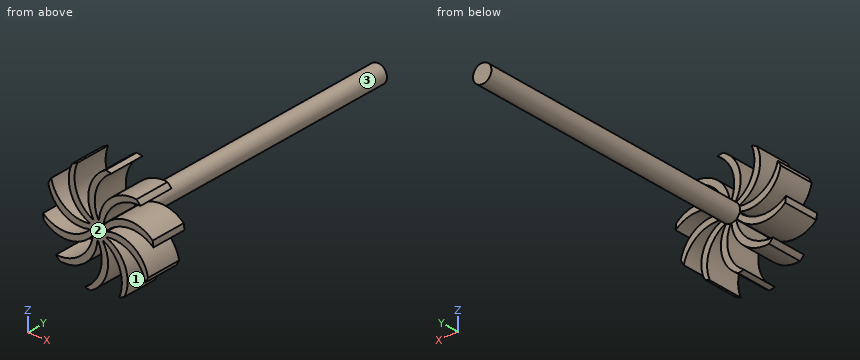
from build123d import *

# Parameters (mm, degrees)
F0_R     = 3.175
F1_DEPTH = 101.6
F3_DEPTH = 12.7


with BuildPart() as f1:
    # F0 (on Front) → F1 (new body)
    with BuildSketch(Plane.XZ):
        Circle(F0_R)
    extrude(amount=F1_DEPTH)

    # F2 (on face) → F3 (join)
    with BuildSketch(Plane.XZ.offset(101.6)):
        with BuildLine():
            ThreePointArc((0, 3.175), (-0.717894, 11.721662), (4.533669, 18.502658))
            ThreePointArc((4.533669, 18.502658), (3.549938, 18.716315), (2.556295, 18.877708))
            ThreePointArc((2.556295, 18.877708), (-3.036137, 11.70738), (-1.6328, 2.722974))
            ThreePointArc((-1.6328, 2.722974), (-0.847108, 3.059907), (0, 3.175))
        make_face()
        with BuildLine():
            ThreePointArc((1.866218, 2.568629), (6.309032, 9.904992), (14.543404, 12.304141))
            ThreePointArc((14.543404, 12.304141), (13.873134, 13.055215), (13.164125, 13.769834))
            ThreePointArc((13.164125, 13.769834), (4.425139, 11.256066), (0.279561, 3.162668))
            ThreePointArc((0.279561, 3.162668), (1.113244, 2.973434), (1.866218, 2.568629))
        make_face()
        with BuildLine():
            ThreePointArc((3.019604, 0.981129), (10.926122, 4.304951), (18.998054, 1.405861))
            ThreePointArc((18.998054, 1.405861), (18.897264, 2.407467), (18.743706, 3.402351))
            ThreePointArc((18.743706, 3.402351), (10.196162, 6.505317), (2.085139, 2.394331))
            ThreePointArc((2.085139, 2.394331), (2.648374, 1.751211), (3.019604, 0.981129))
        make_face()
        with BuildLine():
            ThreePointArc((16.196093, -10.029411), (16.703282, -9.159851), (17.163828, -8.264714))
            ThreePointArc((17.163828, -8.264714), (12.072598, -0.730242), (3.094265, 0.71144))
            ThreePointArc((3.094265, 0.71144), (3.154752, 0.358003), (3.175, 0))
            ThreePointArc((3.175, 0), (3.13591, -0.496679), (3.019604, -0.981129))
            ThreePointArc((3.019604, -0.981129), (11.369805, -2.939435), (16.196093, -10.029411))
        make_face()
        with BuildLine():
            ThreePointArc((-4.533669, -18.502658), (-3.549938, -18.716315), (-2.556295, -18.877708))
            ThreePointArc((-2.556295, -18.877708), (3.036137, -11.70738), (1.6328, -2.722974))
            ThreePointArc((1.6328, -2.722974), (0.847108, -3.059907), (0, -3.175))
            ThreePointArc((0, -3.175), (0.717894, -11.721662), (-4.533669, -18.502658))
        make_face()
        with BuildLine():
            ThreePointArc((7.207774, -17.633788), (8.129213, -17.228418), (9.027952, -16.774939))
            ThreePointArc((9.027952, -16.774939), (9.337711, -7.686873), (2.921487, -1.243196))
            ThreePointArc((2.921487, -1.243196), (2.483893, -1.9776), (1.866218, -2.568629))
            ThreePointArc((1.866218, -2.568629), (7.470609, -9.061056), (7.207774, -17.633788))
        make_face()
        with BuildLine():
            ThreePointArc((-14.543404, -12.304141), (-13.873134, -13.055215), (-13.164125, -13.769834))
            ThreePointArc((-13.164125, -13.769834), (-4.425139, -11.256066), (-0.279561, -3.162668))
            ThreePointArc((-0.279561, -3.162668), (-1.113244, -2.973434), (-1.866218, -2.568629))
            ThreePointArc((-1.866218, -2.568629), (-6.309032, -9.904992), (-14.543404, -12.304141))
        make_face()
        with BuildLine():
            ThreePointArc((-18.998054, -1.405861), (-18.897264, -2.407467), (-18.743706, -3.402351))
            ThreePointArc((-18.743706, -3.402351), (-10.196162, -6.505317), (-2.085139, -2.394331))
            ThreePointArc((-2.085139, -2.394331), (-2.648374, -1.751211), (-3.019604, -0.981129))
            ThreePointArc((-3.019604, -0.981129), (-10.926122, -4.304951), (-18.998054, -1.405861))
        make_face()
        with BuildLine():
            ThreePointArc((-3.019604, 0.981129), (-11.369805, 2.939435), (-16.196093, 10.029411))
            ThreePointArc((-16.196093, 10.029411), (-16.703282, 9.159851), (-17.163828, 8.264714))
            ThreePointArc((-17.163828, 8.264714), (-12.072598, 0.730242), (-3.094265, -0.71144))
            ThreePointArc((-3.094265, -0.71144), (-3.171916, 0.139916), (-3.019604, 0.981129))
        make_face()
        with BuildLine():
            ThreePointArc((-1.866218, 2.568629), (-7.470609, 9.061056), (-7.207774, 17.633788))
            ThreePointArc((-7.207774, 17.633788), (-8.129213, 17.228418), (-9.027952, 16.774939))
            ThreePointArc((-9.027952, 16.774939), (-9.337711, 7.686873), (-2.921487, 1.243196))
            ThreePointArc((-2.921487, 1.243196), (-2.483893, 1.9776), (-1.866218, 2.568629))
        make_face()
        with BuildLine():
            ThreePointArc((3.094265, 0.71144), (3.059907, 0.847108), (3.019604, 0.981129))
            ThreePointArc((3.019604, 0.981129), (2.648374, 1.751211), (2.085139, 2.394331))
            ThreePointArc((2.085139, 2.394331), (1.9776, 2.483893), (1.866218, 2.568629))
            ThreePointArc((1.866218, 2.568629), (1.113244, 2.973434), (0.279561, 3.162668))
            ThreePointArc((0.279561, 3.162668), (0.139916, 3.171916), (0, 3.175))
            ThreePointArc((0, 3.175), (-0.847108, 3.059907), (-1.6328, 2.722974))
            ThreePointArc((-1.6328, 2.722974), (-1.751211, 2.648374), (-1.866218, 2.568629))
            ThreePointArc((-1.866218, 2.568629), (-2.483893, 1.9776), (-2.921487, 1.243196))
            ThreePointArc((-2.921487, 1.243196), (-2.973434, 1.113244), (-3.019604, 0.981129))
            ThreePointArc((-3.019604, 0.981129), (-3.171916, 0.139916), (-3.094265, -0.71144))
            ThreePointArc((-3.094265, -0.71144), (-3.059907, -0.847108), (-3.019604, -0.981129))
            ThreePointArc((-3.019604, -0.981129), (-2.648374, -1.751211), (-2.085139, -2.394331))
            ThreePointArc((-2.085139, -2.394331), (-1.9776, -2.483893), (-1.866218, -2.568629))
            ThreePointArc((-1.866218, -2.568629), (-1.113244, -2.973434), (-0.279561, -3.162668))
            ThreePointArc((-0.279561, -3.162668), (-0.139916, -3.171916), (0, -3.175))
            ThreePointArc((0, -3.175), (0.847108, -3.059907), (1.6328, -2.722974))
            ThreePointArc((1.6328, -2.722974), (1.751211, -2.648374), (1.866218, -2.568629))
            ThreePointArc((1.866218, -2.568629), (2.483893, -1.9776), (2.921487, -1.243196))
            ThreePointArc((2.921487, -1.243196), (2.973434, -1.113244), (3.019604, -0.981129))
            ThreePointArc((3.019604, -0.981129), (3.13591, -0.496679), (3.175, 0))
            ThreePointArc((3.175, 0), (3.154752, 0.358003), (3.094265, 0.71144))
        make_face()
    extrude(amount=F3_DEPTH)


solid = f1.part
For this review, take the finished solid that the model builds, in its own axes (mm). Face numbers are marked on the shaded views. Round coordinates to 2 decimals unless told otherwise and drop trailing zeros. Loops run counter-clockwise (first coordinate to the right, second up) from the corner with the lowest first, then second, coordinate; pieces in that order, holes last. Notation, with made-up numbers: (82, 31.25) - (97, 31.25) arc R12 cw to (97, 50.25) - close; hole circle Ø7 at (20.25, 15). An arc over 180 degrees is marked (long way). Use one line per item in the form item = value.
Item 1: Mouldability with a two-part tool opening along X and no side actions: class the marked faces 1, 2 and 3 as +X half, -X half, draft (parallel to the pull), parting line (faces both ways), or undercut.
Answers:
face_1 = undercut
face_2 = draft
face_3 = parting line
Item 2: For line 1 (Y direction, x = 0, z = 15); line 2 (X direction, y = -104.5, z = 16.5); line 3 (Z direction, x = -1, y = -13.5), list the stretches that pass through material, from the lowest coordinate up.
Answers:
line_1 = -114.3 to -101.6
line_2 = -9.15 to -7.62, -0.46 to 2.04
line_3 = -3.01 to 3.01
Item 3: Clearance check with flat-ended pins moving along their axes: P1, Ø6, axis at x = 13, z = 2.5, coming from the +Y side; P2, Ø10, axis at x = 6.5, y = -56.5, coming from the -Z side; P3, Ø6, axis at x = 8.5, y = -92.5, coming from the +Z side; P4, Ø3, axis at x = -10, y = -101.5, coming from the -Z side. State where each tip first meets the part, or that it passes through.
Answers:
P1 = -101.6
P2 = -2.8
P3 = through
P4 = -13.86
Item 4: Consider section A-A on z = -15. Write out the cut boundary in (x, y), then the cut area to 3 significant figures.
Answers:
outline = (-0.83, -114.3) - (1.6, -114.3) - (1.6, -101.6) - (-0.83, -101.6) - close; (7.98, -114.3) - (9.7, -114.3) - (9.7, -101.6) - (7.98, -101.6) - close
area = 52.7 mm^2
Item 5: Consider section B-B on y = -23. Write out the cut boundary in (x, z) (3 decimals), then the cut area to 3 significant figures.
Answers:
outline = circle Ø6.35 at (0, 0)
area = 31.7 mm^2
